Geometry: final body of the model. Coordinates: model frame, mm. A direction names the side the tool comes from. Give positions to 0.01 mm unless a question says otherwise; leave off trailing zeros. Write each loop counter-clockwise with the first axis right and the second up, starting at its lowest first coordinate (ties: lowest second). Pieces come first, ordered by that corner, then holes. Notation, with made-up numbers: (74.25, 68.5) - (116.25, 68.5) arc R27 cw to (116.25, 97.5) - close; hole circle Ø9 at (-2, 33.25). An arc over 180 degrees is marked (long way). One line per question, with ' | ' between items. Start each with the question number.
```python
from build123d import *
from OCP.BRepFilletAPI import BRepFilletAPI_MakeChamfer

# Parameters (mm, degrees)
SKETCH1_W           = 380
SKETCH1_H           = 400
BOSS_EXTRUDE1_DEPTH = 85
SKETCH2_W           = 80
SKETCH2_H           = 390
BOSS_EXTRUDE2_DEPTH = 150
CHAMFER1_SIZE       = 72.794046853
CHAMFER1_SIZE_2     = 200
CHAMFER2_SIZE       = 130
CHAMFER2_SIZE2      = 47.316130455
SKETCH3_W           = 380
SKETCH3_H           = 600
BOSS_EXTRUDE3_DEPTH = 50
SKETCH4_R           = 50
BOSS_EXTRUDE4_DEPTH = 300


with BuildPart() as part:
    # Sketch1 → Boss-Extrude1 (new body)
    with BuildSketch(Plane(origin=(0, 0, 0), x_dir=(1, 0, 0), z_dir=(0, 1, 0))):
        Rectangle(SKETCH1_W, SKETCH1_H)
    extrude(amount=BOSS_EXTRUDE1_DEPTH)

    # Sketch2 → Boss-Extrude2 (add)
    with BuildSketch(Plane(origin=(0, 0, 0), x_dir=(1, 0, 0), z_dir=(0, 1, 0))):
        with Locations((-230, 0)):
            Rectangle(SKETCH2_W, SKETCH2_H)
        with Locations((230, 0)):
            Rectangle(SKETCH2_W, SKETCH2_H)
    extrude(amount=BOSS_EXTRUDE2_DEPTH)

    # Chamfer1
    # the kernel refuses this chamfer: 200, 72.794046853 mm, written as the material it takes off along each edge
    with BuildSketch(Plane(origin=(-788.83894651, 150, 195), x_dir=(0, -0.9950833631817488, 0.09904090225204945), z_dir=(1, 0, 0)), Plane(origin=(190, 150, 195), x_dir=(0, -0.9950833631817488, 0.09904090225204945), z_dir=(1, 0, 0))) as chamfer1_piece_1:
        Polygon((CHAMFER1_SIZE * 0.995083363185, CHAMFER1_SIZE * 0.0990409022524), (-CHAMFER1_SIZE_2 * 0.099040902252, CHAMFER1_SIZE_2 * 0.995083363182), (0, 0), align=None)
    extrude(amount=598.83894651, mode=Mode.SUBTRACT)
    with BuildSketch(Plane(origin=(-788.83894651, 150, 195), x_dir=(0, -0.9950833631817488, 0.09904090225204945), z_dir=(1, 0, 0))) as chamfer1_piece_2_section:
        Polygon((CHAMFER1_SIZE * 0.995083363185, CHAMFER1_SIZE * 0.0990409022524), (-CHAMFER1_SIZE_2 * 0.099040902252, CHAMFER1_SIZE_2 * 0.995083363182), (0, 0), align=None)
    chamfer1_piece_2 = extrude(amount=1117.67789302, mode=Mode.PRIVATE)
    chamfer1_piece_2 = split(chamfer1_piece_2, bisect_by=Plane(origin=(190, 82.401984382, 187.862010755), z_dir=(1, 0, 0)), keep=Keep.TOP, mode=Mode.PRIVATE)
    add(chamfer1_piece_2, mode=Mode.SUBTRACT)
    with BuildSketch(Plane(origin=(-328.83894651, 150, 195), x_dir=(0, -0.9950833631817488, 0.09904090225204945), z_dir=(1, 0, 0))) as chamfer1_piece_3_section:
        Polygon((CHAMFER1_SIZE * 0.995083363185, CHAMFER1_SIZE * 0.0990409022524), (-CHAMFER1_SIZE_2 * 0.099040902252, CHAMFER1_SIZE_2 * 0.995083363182), (0, 0), align=None)
    chamfer1_piece_3 = extrude(amount=1117.67789302, mode=Mode.PRIVATE)
    chamfer1_piece_3 = split(chamfer1_piece_3, bisect_by=Plane(origin=(-190, 82.401984382, 187.862010755), z_dir=(-1, 0, 0)), keep=Keep.TOP, mode=Mode.PRIVATE)
    add(chamfer1_piece_3, mode=Mode.SUBTRACT)

    # Chamfer2: one chamfer whose edges measure the first distance from different faces: ONE call of the kernel's chamfer builder (chamfer() names one face for all edges)
    chamfer2_edges_1 = [part.edges().sort_by_distance(p)[0] for p in [
        (270, 0, 0),
    ]]
    chamfer2_side_1 = [part.faces().sort_by_distance(p)[0] for p in [
        (270, 67.789562339, -18.238567166),
    ]]
    chamfer2_edges_2 = [part.edges().sort_by_distance(p)[0] for p in [
        (-270, 0, 0),
    ]]
    chamfer2_side_2 = [part.faces().sort_by_distance(p)[0] for p in [
        (-270, 67.789562339, -18.238567166),
    ]]
    chamfer2 = BRepFilletAPI_MakeChamfer(part.part.solid().wrapped)
    for e in chamfer2_edges_1:
        chamfer2.Add(CHAMFER2_SIZE, CHAMFER2_SIZE2, e.wrapped, chamfer2_side_1[0].wrapped)  # the first distance lies on this face
    for e in chamfer2_edges_2:
        chamfer2.Add(CHAMFER2_SIZE, CHAMFER2_SIZE2, e.wrapped, chamfer2_side_2[0].wrapped)  # the first distance lies on this face
    add(Compound.cast(chamfer2.Shape()), mode=Mode.REPLACE)

    # Sketch3 → Boss-Extrude3 (add)
    with BuildSketch(Plane(origin=(0, 0, -200), x_dir=(-1, 0, 0), z_dir=(0, 0, -1))):
        with Locations((0, 300)):
            Rectangle(SKETCH3_W, SKETCH3_H)
    extrude(amount=BOSS_EXTRUDE3_DEPTH)

    # Sketch4 → Boss-Extrude4 (add)
    with BuildSketch(Plane.XZ):
        with Locations(Location((0, 0, 0), (0, 0, 270))):
            Circle(SKETCH4_R)
    extrude(amount=BOSS_EXTRUDE4_DEPTH)


solid = part.part
```
1) Line query: L1, parallel to Z at x = 25.5, y = 410; L2, parallel to Y at x = 58, z = -80; L3, parallel to X at y = 211, z = -206. Output: solid intervals per line, ascending.
2) First-contact query: pin 1 Ø8 at (y, z) = (36.5, 191) entering from +X; pin 2 Ø19.5 at (y, z) = (131.5, 70) entering from +X; pin 3 Ø18 at (x, y) = (-228, 31.5) entering from +Z. Flat tips, straight axial feed; report the tip coordinate or a pass-through.
3) Reachability of faces 1 (the flat face through (-222, 91, -195)), 2 (the flat face through (-190, 117, -49)), 3 (the flat face through (-190, 49, 197)), 4 (the flat face through (213, 38, 195)), 5 (the flat face through (190, 49, 197)) from +Z, -Z, +X, -X, +Y, -Y: full face, straight path, thin tool, end or side. Return the list, or none.
4) Section B-B, the plane z = 104. Output: boundary loops of the cut face in (x, y).
5) Section C-C, the plane y = 401. Output: boundary loops of the cut face in (x, z), plus the area to 3 significant figures.
6) Section A-A, the plane x = -116.5. Output: boundary loops of the cut face in (y, z).
7) Pull-direction query (X, two-part tool) for faces 6 (the flat face through (-190, 296, -222)), 7 (the flat face through (221, 91, -195)), 8 (the flat face through (190, 117, -49)); classes: +X half, -X half, draft (parallel to the pull), parting line (faces both ways), or undercut.
8) Section D-D, the plane x = 0. Output: boundary loops of the cut face in (y, z).
Answer key:
1) L1: -250 to -200 | L2: 0 to 85 | L3: -190 to 190
2) pin 1: x = 237.42 | pin 2: x = 268.36 | pin 3: z = 195
3) face 1: -Z, -X, +Y, -Y | face 2: +Z, +Y | face 3: +Z, -X, +Y | face 4: +Z, +X, +Y, -Y | face 5: +Z, +X, +Y
4) outline: (-262.84, 110.33) - (-222.68, 0) - (222.68, 0) - (262.84, 110.33) - (190, 110.33) - (190, 85) - (-190, 85) - (-190, 110.33) - close
5) outline: (-190, -250) - (190, -250) - (190, -200) - (-190, -200) - close | area: 19,000 mm^2
6) outline: (0, -250) - (600, -250) - (600, -200) - (85, -200) - (85, 200) - (0, 200) - close
7) face 6: -X half | face 7: draft | face 8: undercut
8) outline: (-300, -50) - (0, -50) - (0, -250) - (600, -250) - (600, -200) - (85, -200) - (85, 200) - (0, 200) - (0, 50) - (-300, 50) - close
